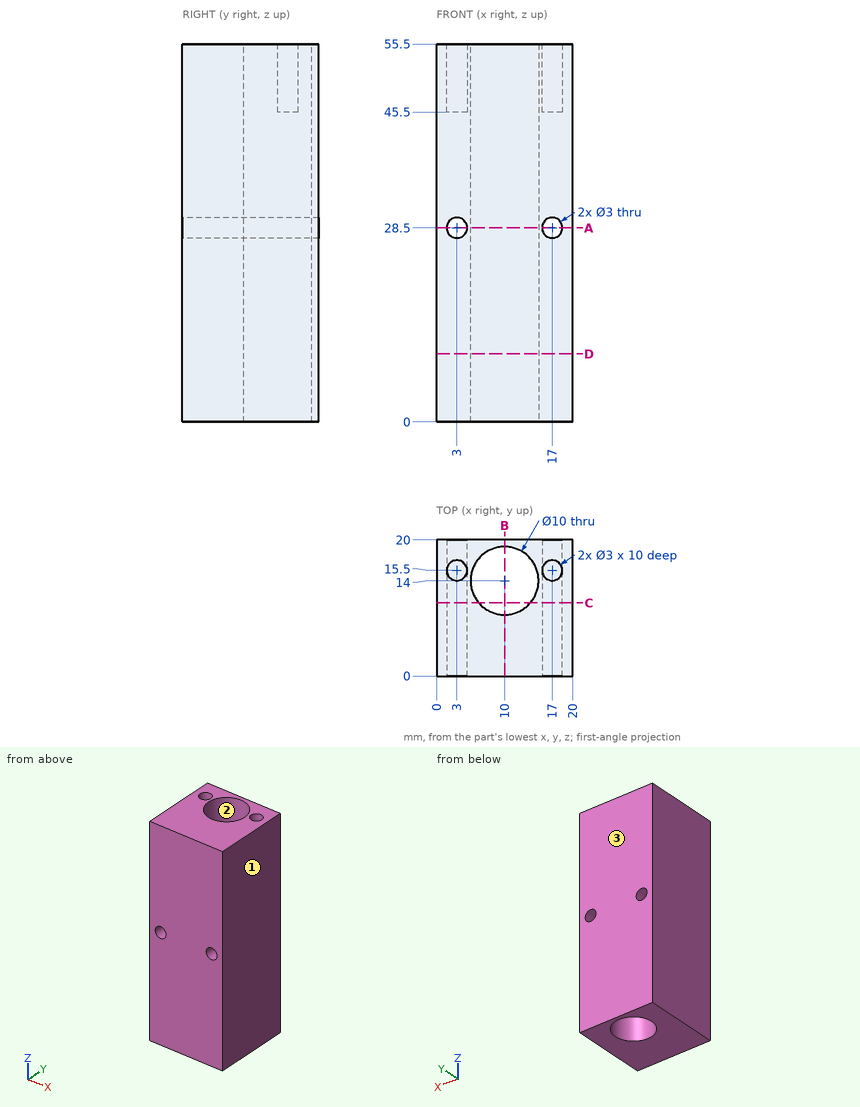
The figure shows three views and two pictorial views of one solid part (mm, origin at its lowest corner). Answer the questions. Give positions to 0.01 mm unless a question says otherwise; leave off trailing zeros. Order: outer loops, then holes, each group sorted by start corner. A loop starts at its lowest first (then second) coordinate and runs counter-clockwise, first axis right, second up. Notation, with made-up numbers: (17.25, -18) -> (30.25, -18) arc R13 ccw to (30.25, -3) -> close; hole circle Ø6 at (6.5, 22.5). An arc over 180 degrees is marked (long way). Answer as a JSON object with one key per item and string values. Group by question number.
Item 1: Consider L1, parallel to Y at x = 17, z = 47.5; L2, parallel to Y at x = 10, z = 39; L3, parallel to X at y = 15.75, z = 14. Determine where each line is inside the solid, lowest interval first. Write a range as from..to.
Item 2: Flat-ended cylindrical pins translate along their axes: pin 1 (5 mm diameter, centred on y = 9.5, z = 36.5, fed in from -X); pin 2 (1.5 mm diameter, centred on x = 16.5, y = 16, fed in from +Z). Find the tip coordinate at first contact, or state that the pin passes through.
Item 3: The part is cut by section D-D on z = 10. Write down the section's boundary in (x, y).
Item 4: Determine the mould class of the marked faces 1, 2 and 3 for opening direction Y: pulls with the +Y half, pulls with the -Y half, needs draft (parallel to the pull), parting line crosses it, or undercut.
Item 5: The part is cut by section C-C on y = 10.75. Write down the section's boundary in (x, z), and give its area (3 significant figures).
Item 6: The part is cut by section B-B on x = 10. Write down the section's boundary in (y, z), and give its area (3 significant figures).
Item 7: The part is cut by section A-A on z = 28.5. Write down the section's boundary in (x, y), and give its area (3 significant figures).
Result set:
{
 "1": {"L1": "0..14, 17..20", "L2": "0..9, 19..20", "L3": "0..5.32, 14.68..20"},
 "2": {"pin 1": "x = 0", "pin 2": "z = 45.5"},
 "3": {"outline": "(0, 0) -> (20, 0) -> (20, 20) -> (0, 20) -> close; hole circle Ø10 at (10, 14)"},
 "4": {"face 1": "needs draft", "face 2": "undercut", "face 3": "pulls with the +Y half"},
 "5": {"outline": "(0, 0) -> (6.2, 0) -> (6.2, 55.5) -> (0, 55.5) -> close; (13.8, 0) -> (20, 0) -> (20, 55.5) -> (13.8, 55.5) -> close; hole circle Ø3 at (3, 28.5); hole circle Ø3 at (17, 28.5)", "area": "674 mm²"},
 "6": {"outline": "(0, 0) -> (9, 0) -> (9, 55.5) -> (0, 55.5) -> close; (19, 0) -> (20, 0) -> (20, 55.5) -> (19, 55.5) -> close", "area": "555 mm²"},
 "7": {"outline": "(0, 0) -> (1.5, 0) -> (1.5, 20) -> (0, 20) -> close; (4.5, 0) -> (15.5, 0) -> (15.5, 20) -> (4.5, 20) -> close; (18.5, 0) -> (20, 0) -> (20, 20) -> (18.5, 20) -> close; hole circle Ø10 at (10, 14)", "area": "201 mm²"}
}
